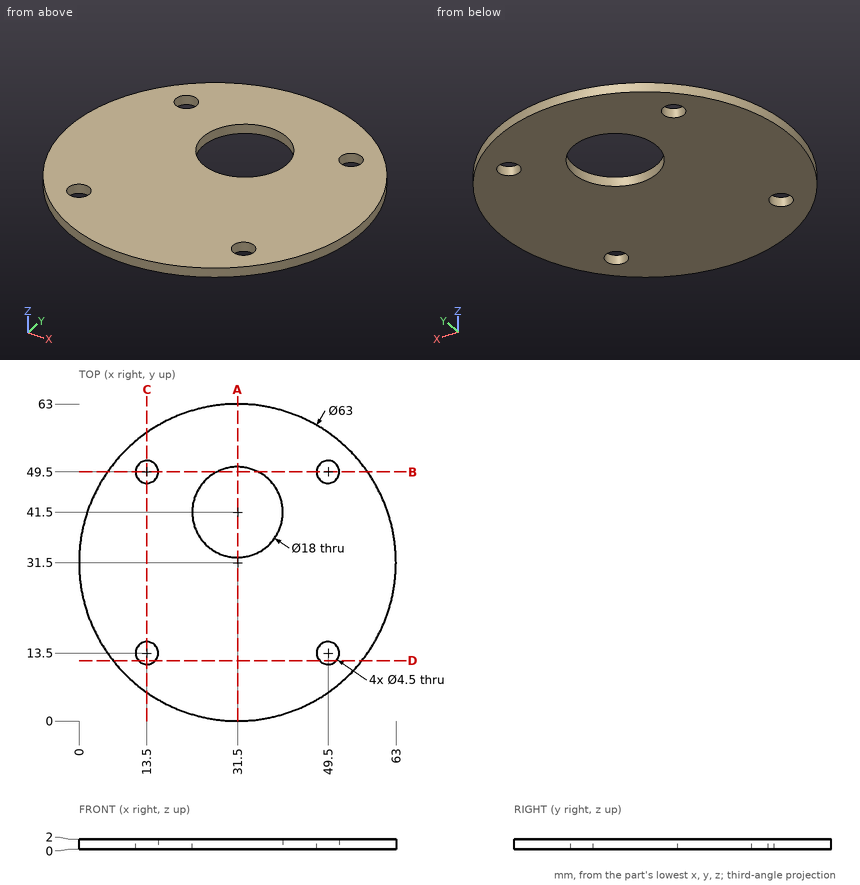
Geometry check sheet. Reference: drawing and pictorial views, mm from the part's lowest x, y, z. Coordinates: 2 decimals unless noted, no trailing zeros. Write each loop counter-clockwise with the first axis right and the second up, starting at its lowest first coordinate (ties: lowest second). Pieces come first, ordered by that corner, then holes. Notation, with made-up numbers: M -1,16.25 L 17,16.25 A20 cw 17,40.25 Z; hole C 57.5,-35 d11. An arc over 180 degrees is marked long. Use one line per item in the form item = value.
Item 1: Sectioned sample at D-D, the plane y = 12. Record the cut outline in (x, z).
Answer below:
outline = M 6.76,0 L 11.82,0 L 11.82,2 L 6.76,2 Z; M 15.18,0 L 47.82,0 L 47.82,2 L 15.18,2 Z; M 51.18,0 L 56.24,0 L 56.24,2 L 51.18,2 Z
Item 2: Sectioned sample at C-C, the plane x = 13.5. Record the cut outline in (y, z), and give its area (3 significant figures).
Answer below:
outline = M 5.65,0 L 11.25,0 L 11.25,2 L 5.65,2 Z; M 15.75,0 L 47.25,0 L 47.25,2 L 15.75,2 Z; M 51.75,0 L 57.35,0 L 57.35,2 L 51.75,2 Z
area = 85.4 mm^2
Item 3: Sectioned sample at A-A, the plane x = 31.5. Record the cut outline in (y, z).
Answer below:
outline = M 0,0 L 32.5,0 L 32.5,2 L 0,2 Z; M 50.5,0 L 63,0 L 63,2 L 50.5,2 Z
Item 4: Sectioned sample at B-B, the plane y = 49.5. Record the cut outline in (x, z), and give its area (3 significant figures).
Answer below:
outline = M 5.65,0 L 11.25,0 L 11.25,2 L 5.65,2 Z; M 15.75,0 L 27.38,0 L 27.38,2 L 15.75,2 Z; M 35.62,0 L 47.25,0 L 47.25,2 L 35.62,2 Z; M 51.75,0 L 57.35,0 L 57.35,2 L 51.75,2 Z
area = 68.9 mm^2
Item 5: Material ranges on L1, parallel to Y at x = 13.5, z = 0.7; L2, parallel to X at y = 13, z = 1.4; L3, parallel to Y at x = 31.5, z = 1.65, recorded low to high. Write a range as from..to.
Answer below:
L1 = 5.65..11.25, 15.75..47.25, 51.75..57.35
L2 = 6..11.31, 15.69..47.31, 51.69..57
L3 = 0..32.5, 50.5..63
